```python
from build123d import *

# Parameters (mm, degrees)
SKETCH2_W           = 26
SKETCH2_H           = 11.2
BOSS_EXTRUDE1_DEPTH = 20
SKETCH6_W           = 14
SKETCH6_H           = 2.4
CUT_EXTRUDE1_DEPTH  = 20
SKETCH7_W           = 10.08
SKETCH7_H           = 4.9
CUT_EXTRUDE2_DEPTH  = 15
SKETCH8_W           = 19
SKETCH8_H           = 1.78
CUT_EXTRUDE3_DEPTH  = 16
SKETCH9_W           = 15.8
SKETCH9_H           = 2.12
CUT_EXTRUDE4_DEPTH  = 15
SKETCH10_W          = 3
SKETCH10_H          = 2
CUT_EXTRUDE5_DEPTH  = 15
CUT_REVOLVE3_ANGLE  = 180
SKETCH15_W          = 12
SKETCH15_H          = 6
BOSS_EXTRUDE2_DEPTH = 10
SKETCH16_W          = 12
SKETCH16_H          = 6
BOSS_EXTRUDE3_DEPTH = 10
SKETCH17_R          = 2
CUT_EXTRUDE6_DEPTH  = 12
SKETCH18_R          = 2
CUT_EXTRUDE7_DEPTH  = 12


with BuildPart() as part:
    # Sketch2 → Boss-Extrude1 (new body)
    with BuildSketch(Plane.XY):
        Rectangle(SKETCH2_W, SKETCH2_H)
    extrude(amount=BOSS_EXTRUDE1_DEPTH)

    # Sketch6 → Cut-Extrude1 (cut)
    with BuildSketch(Plane.XY.offset(20)):
        with Locations((0, -4.4)):
            Rectangle(SKETCH6_W, SKETCH6_H)
    extrude(amount=-CUT_EXTRUDE1_DEPTH, mode=Mode.SUBTRACT)

    # Sketch7 → Cut-Extrude2 (cut)
    with BuildSketch(Plane.XY.offset(20)):
        with Locations((0, -0.75)):
            Rectangle(SKETCH7_W, SKETCH7_H)
    extrude(amount=-CUT_EXTRUDE2_DEPTH, mode=Mode.SUBTRACT)

    # Sketch8 → Cut-Extrude3 (cut)
    with BuildSketch(Plane.XY.offset(20)):
        with Locations((2.3, 2.59)):
            Rectangle(SKETCH8_W, SKETCH8_H)
    extrude(amount=-CUT_EXTRUDE3_DEPTH, mode=Mode.SUBTRACT)

    # Sketch9 → Cut-Extrude4 (cut)
    with BuildSketch(Plane.XY.offset(20)):
        with Locations((2.7, 4.54)):
            Rectangle(SKETCH9_W, SKETCH9_H)
    extrude(amount=-CUT_EXTRUDE4_DEPTH, mode=Mode.SUBTRACT)

    # Sketch10 → Cut-Extrude5 (cut)
    with BuildSketch(Plane.XY.offset(20)):
        with Locations((9.1, 0.7)):
            Rectangle(SKETCH10_W, SKETCH10_H)
    extrude(amount=-CUT_EXTRUDE5_DEPTH, mode=Mode.SUBTRACT)

    # Sketch11 → Cut-Revolve3 (revolve, cut)
    with BuildSketch(Plane.XZ.offset(5.6)):
        with BuildLine():
            Line((-11.55, 5), (-8.45, 5))
            ThreePointArc((-8.45, 5), (-10, 6.55), (-11.55, 5))
        make_face()
    revolve(axis=Axis((-11.55, -5.6, 5), (-1, 0, 0)), revolution_arc=CUT_REVOLVE3_ANGLE, mode=Mode.SUBTRACT)

    # Sketch12 → Revolve2 (revolve)
    with BuildSketch(Plane.XZ.offset(5.6)):
        with BuildLine():
            Line((-11.5, 15), (-8.5, 15))
            ThreePointArc((-8.5, 15), (-10, 13.5), (-11.5, 15))
        make_face()
    revolve(axis=Axis((-11.5, -5.6, 15), (1, 0, 0)))

    # Sketch14 → Cut-Revolve4 (revolve, cut)
    with BuildSketch(Plane.XZ.offset(5.6)):
        with BuildLine():
            Line((8.45, 15), (11.55, 15))
            ThreePointArc((11.55, 15), (10, 13.45), (8.45, 15))
        make_face()
    revolve(axis=Axis((8.45, -5.6, 15), (1, 0, 0)), mode=Mode.SUBTRACT)

    # Sketch13 → Revolve3 (revolve)
    with BuildSketch(Plane.XZ.offset(5.6)):
        with BuildLine():
            Line((8.5, 5), (11.5, 5))
            ThreePointArc((11.5, 5), (10, 6.5), (8.5, 5))
        make_face()
    revolve(axis=Axis((8.5, -5.6, 5), (1, 0, 0)))

    # Sketch15 → Boss-Extrude2 (add)
    with BuildSketch(Plane.ZY.offset(13)):
        with Locations((6, -2.6)):
            Rectangle(SKETCH15_W, SKETCH15_H)
    extrude(amount=BOSS_EXTRUDE2_DEPTH)

    # Sketch16 → Boss-Extrude3 (add)
    with BuildSketch(Plane(origin=(13, 0, 0), x_dir=(0, 0, -1), z_dir=(1, 0, 0))):
        with Locations((-6, -2.6)):
            Rectangle(SKETCH16_W, SKETCH16_H)
    extrude(amount=BOSS_EXTRUDE3_DEPTH)

    # Sketch17 → Cut-Extrude6 (cut)
    with BuildSketch(Plane.XZ.offset(5.6)):
        with Locations(Location((-18, 6, 0), (0, 0, 270))):
            Circle(SKETCH17_R)
    extrude(amount=-CUT_EXTRUDE6_DEPTH, mode=Mode.SUBTRACT)

    # Sketch18 → Cut-Extrude7 (cut)
    with BuildSketch(Plane.XZ.offset(5.6)):
        with Locations(Location((18, 6, 0), (0, 0, 270))):
            Circle(SKETCH18_R)
    extrude(amount=-CUT_EXTRUDE7_DEPTH, mode=Mode.SUBTRACT)


solid = part.part
```
Design review of the part built by this model. Coordinates are the model's own, in mm. A direction names the side the tool comes from. Give positions to 0.01 mm unless a question says otherwise; leave off trailing zeros. Write each loop counter-clockwise with the first axis right and the second up, starting at its lowest first coordinate (ties: lowest second). Pieces come first, ordered by that corner, then holes. Notation, with made-up numbers: (-24, 36.5) -> (32, 36.5) arc R13 ccw to (32, 41.5) -> close; hole circle Ø10 at (24, 9.5). An arc over 180 degrees is marked (long way). Answer in a Markdown table with one row per item.
(1) For faces 5 (the flat face through (6, 1.7, 10)), 6 (the flat face through (-18, -3, 12)), 7 (the flat face through (18, -3, 12)), 8 (the flat face through (20.2, 0.4, 6.1)), 9 (the flat face through (9, 1, 5)), list the 3-axis set-ups (+Z, -Z, +X, -X, +Y, -Y) from which the entire face can be reached by the end or side of a thin tool; tool diameter is ignored.
Results:
| item | result |
|---|---|
| face 5 | +Z |
| face 6 | +Z, -X, +Y, -Y |
| face 7 | +Z, +X, +Y, -Y |
| face 8 | +Z, -Z, +X, +Y |
| face 9 | +Z, +Y |
(2) Consider section A-A (z = 17.25). State the section outline as (x, y) points.
Results:
| item | result |
|---|---|
| outline | (-13, -5.6) -> (-7, -5.6) -> (-7, -3.2) -> (-5.04, -3.2) -> (-5.04, 1.7) -> (-7.2, 1.7) -> (-7.2, 3.48) -> (-5.2, 3.48) -> (-5.2, 5.6) -> (-13, 5.6) -> close; (5.04, -3.2) -> (7, -3.2) -> (7, -5.6) -> (13, -5.6) -> (13, 5.6) -> (10.6, 5.6) -> (10.6, 3.48) -> (11.8, 3.48) -> (11.8, 1.7) -> (10.6, 1.7) -> (10.6, -0.3) -> (7.6, -0.3) -> (7.6, 1.7) -> (5.04, 1.7) -> close |
(3) Clearance check with flat-ended pins moving along their axes: pin 1 (6.5 mm diameter, centred on x = 18, z = 6, fed in from -Y); pin 2 (1.5 mm diameter, centred on y = 3.5, z = 3, fed in from -X); pin 3 (6 mm diameter, centred on x = 3.5, y = 2.5, fed in from -Z); pin 4 (0.9 mm diameter, centred on x = 0.5, y = 3, fed in from +Z). State where each tip first meets the part, or that it passes through.
Results:
| item | result |
|---|---|
| pin 1 | y = -5.6 |
| pin 2 | x = -13 |
| pin 3 | z = 0 |
| pin 4 | z = 4 |
(4) Consider section D-D (y = 4). State the section outline as (x, z) points.
Results:
| item | result |
|---|---|
| outline | (-13, 0) -> (13, 0) -> (13, 20) -> (10.6, 20) -> (10.6, 5) -> (-5.2, 5) -> (-5.2, 20) -> (-13, 20) -> close |
(5) Consider section C-C (y = -2). State the section outline as (x, z) points.
Results:
| item | result |
|---|---|
| outline | (-23, 0) -> (23, 0) -> (23, 12) -> (13, 12) -> (13, 20) -> (5.04, 20) -> (5.04, 5) -> (-5.04, 5) -> (-5.04, 20) -> (-13, 20) -> (-13, 12) -> (-23, 12) -> close; hole circle Ø4 at (-18, 6); hole circle Ø4 at (18, 6) |
(6) Consider section B-B (x = -18). State the section outline as (y, z) points.
Results:
| item | result |
|---|---|
| outline | (-5.6, 0) -> (0.4, 0) -> (0.4, 4) -> (-5.6, 4) -> close; (-5.6, 8) -> (0.4, 8) -> (0.4, 12) -> (-5.6, 12) -> close |
(7) To check wall thickness, follow probe 1 along X at (y, z) = (1.25, 10.25); probe 2 along X at (y, z) = (-0.9, 6); probe 3 along X at (y, z) = (-3, 5.25). State the ranges of each line that lie inside material, in increasing order.
Results:
| item | result |
|---|---|
| probe 1 | -13 to -5.04, 5.04 to 7.6, 10.6 to 13 |
| probe 2 | -23 to -20, -16 to -5.04, 5.04 to 16, 20 to 23 |
| probe 3 | -23 to -19.85, -16.15 to -5.04, 5.04 to 16.15, 19.85 to 23 |
(8) Mouldability with a two-part tool opening along X and no side actions: class faces 1 (the flat face through (23, -3, 6)), 2 (the flat face through (-23, -3, 6)), 3 (the flat face through (0, 0, 0)), 4 (the flat face through (-5.04, -1, 13)) as +X half, -X half, draft (parallel to the pull), parting line (faces both ways), or undercut.
Results:
| item | result |
|---|---|
| face 1 | +X half |
| face 2 | -X half |
| face 3 | draft |
| face 4 | undercut |
